Geometry check sheet. Reference: drawing and pictorial views, mm from the part's lowest x, y, z. A direction names the side the tool comes from. Give positions to 0.01 mm unless a question says otherwise; leave off trailing zeros. Write each loop counter-clockwise with the first axis right and the second up, starting at its lowest first coordinate (ties: lowest second). Pieces come first, ordered by that corner, then holes. Notation, with made-up numbers: M -36.75,56 L 2.25,56 A23 cw 2.25,69 Z; hole C 76,42.25 d2. An arc over 180 degrees is marked long. Write item = value, one per line. Start each with the question number.
1) Mould release check, pull along Y, two halves, no side actions. Record for the marked faces 3, 4 and 5: released by +Y, released by -Y, zero draft, split by the parting line, or undercut.
2) Go/stop test with a flat-tipped pin: pin 1 (8 mm diameter, centred on y = 169, z = 27.5, fed in from +X). Record where the tip stops, or that it passes through.
3) Cross-section at A-A, the plane z = 76. Record the cut outline in (x, y).
4) Cross-section at D-D, the plane z = 43. Record the cut outline in (x, y), plus the area to 3 significant figures.
5) Access from +Z, -Z, +X, -X, +Y, -Y to the whole of each face (thin tool, end or side, straight path). Record for the marked faces 1 and 2.
6) Cross-section at B-B, the plane x = 179.5. Record the cut outline in (y, z), plus the area to 3 significant figures.
7) Scan lines: line 1 along Y through (x, z) = (210, 24); line 2 along Y through (x, z) = (230, 87); line 3 along X through (y, z) = (18.5, 64). Record each from-to range of solid material in increasing order. Write a range as [from, to].
8) Cross-section at C-C, the plane y = 151. Record the cut outline in (x, z).
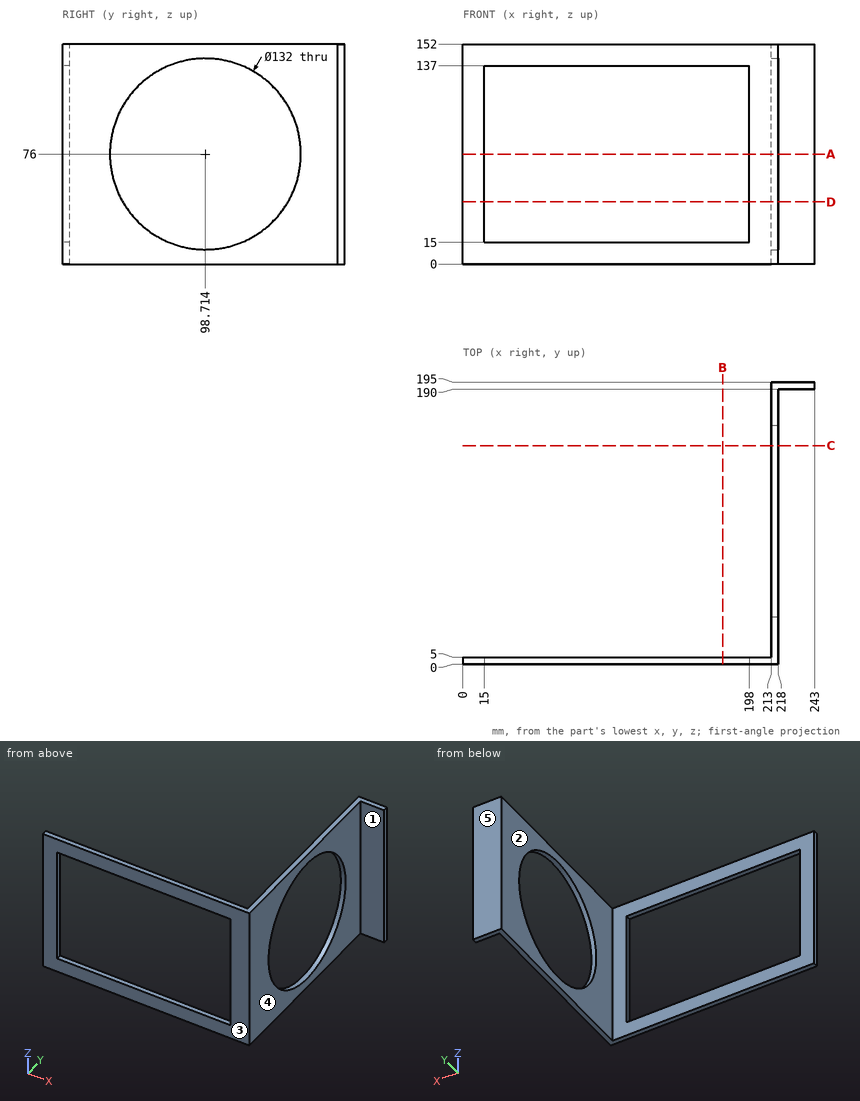
Reply:
q1.face_3 = released by -Y
q1.face_4 = zero draft
q1.face_5 = released by +Y
q2.pin_1 = 218
q3.outline = M 0,0 L 15,0 L 15,5 L 0,5 Z; M 198,0 L 218,0 L 218,32.71 L 213,32.71 L 213,5 L 198,5 Z; M 213,164.71 L 218,164.71 L 218,190 L 243,190 L 243,195 L 213,195 Z
q4.outline = M 0,0 L 15,0 L 15,5 L 0,5 Z; M 198,0 L 218,0 L 218,41.56 L 213,41.56 L 213,5 L 198,5 Z; M 213,155.87 L 218,155.87 L 218,190 L 243,190 L 243,195 L 213,195 Z
q4.area = 678 mm2
q5.face_1 = +Z, -Z, +X, -Y
q5.face_2 = +Z, -Z, -X, +Y
q6.outline = M 0,0 L 5,0 L 5,15 L 0,15 Z; M 0,137 L 5,137 L 5,152 L 0,152 Z
q6.area = 150 mm2
q7.line_1 = [0, 5]
q7.line_2 = [190, 195]
q7.line_3 = [213, 218]
q8.outline = M 213,0 L 218,0 L 218,35.72 L 213,35.72 Z; M 213,116.28 L 218,116.28 L 218,152 L 213,152 Z
